from build123d import *

# Parameters (mm, degrees)
F2_SIZE  = 0.381
F4_DEPTH = 25.019
F5_R     = 6.875
F6_DEPTH = 25.781


with BuildPart() as f1:
    # F0 (on Front) → F1 (revolve)
    with BuildSketch(Plane.XZ):
        Polygon((22.225, 12.7), (-22.225, 12.7), (-22.225, 31.75), (-25.4, 31.75), (-25.4, 0), (25.4, 0), (25.4, 31.75), (22.225, 31.75), align=None)
    revolve(axis=Axis((0, 0, 0), (1, 0, 0)))

    # F2
    f2_edges = [f1.edges().sort_by_distance(p)[0] for p in [
        (-22.225, 0, -31.75),
        (-25.4, 0, -31.75),
        (22.225, 0, -31.75),
        (25.4, 0, -31.75),
    ]]
    chamfer(f2_edges, length=F2_SIZE)

    # F3 (on face) → F4 (cut)
    with BuildSketch(Plane.YZ.offset(25.4)):
        Polygon((6.35, -3.666174), (6.35, 3.666174), (0, 7.332348), (-6.35, 3.666174), (-6.35, -3.666174), (0, -7.332348), align=None)
    extrude(amount=-F4_DEPTH, mode=Mode.SUBTRACT)

    # F5 (on face) → F6 (cut)
    with BuildSketch(Plane(origin=(-25.4, 0, 0), x_dir=(0, -1, 0), z_dir=(-1, 0, 0))):
        Circle(F5_R)
    extrude(amount=-F6_DEPTH, mode=Mode.SUBTRACT)


solid = f1.part
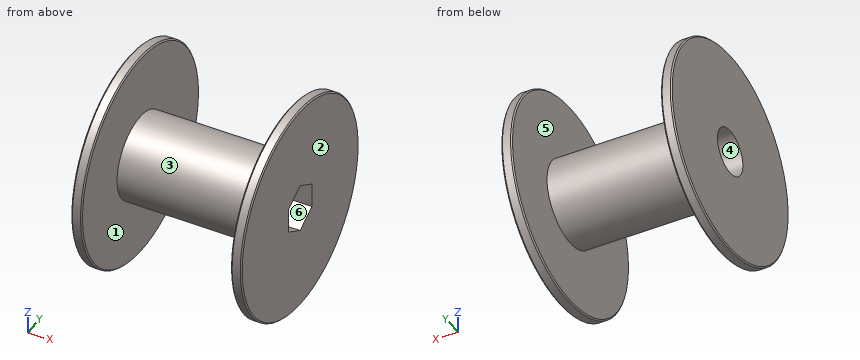
Geometry: final body of the model. Coordinates: model frame, mm. Face numbers are marked on the shaded views. A direction names the side the tool comes from. Round coordinates to 2 decimals unless told otherwise and drop trailing zeros. Order: outer loops, then holes, each group sorted by start corner. A loop starts at its lowest first (then second) coordinate and runs counter-clockwise, first axis right, second up. Notation, with made-up numbers: (15, 69) -> (67, 69) arc R27 ccw to (67, 95) -> close; hole circle Ø8 at (2.5, 38.25). An arc over 180 degrees is marked (long way). Put each result on its own line as item: value. Start each with the question number.
Q1. Line query: probe 1 along Y at (x, z) = (-7, 0) (3 decimals); probe 2 along X at (y, z) = (15, -2) (3 decimals). Output: solid intervals per line, ascending.
Q2. Section B-B on x = 13. Return the cut outline in (y, z), and give its area (3 significant figures).
Q3. First-contact query: pin 1 (8 mm diameter, centred on x = 14.5, y = -13.5, fed in from +Z); pin 2 (10 mm diameter, centred on x = -16.5, y = -6, fed in from +Z); pin 3 (2 mm diameter, centred on x = 8.5, z = 5.5, fed in from -Y). Flat tips, straight axial feed; report the tip coordinate or a pass-through.
Q4. Section C-C on x = -13.5. Return the cut outline in (y, z) (3 decimals).
Q5. Section A-A on z = 0. Return the cut outline in (x, y) (3 decimals), and give its area (3 significant figures).
Q6. Reachability of the marked faces 1 and 2 from +Z, -Z, +X, -X, +Y, -Y: full face, straight path, thin tool, end or side. Return the list, or none.
Q7. Pull-direction query (Z, two-part tool) for the marked faces 3, 4, 5 and 6; classes: +Z half, -Z half, draft (parallel to the pull), parting line (faces both ways), or undercut.
Ans:
1. probe 1: y = -12.7 to -6.875, 6.875 to 12.7
1. probe 2: x = -25.4 to -22.225, 22.225 to 25.4
2. outline: circle Ø25.4 at (0, 0); hole (-6.35, -3.67) -> (0, -7.33) -> (6.35, -3.67) -> (6.35, 3.67) -> (0, 7.33) -> (-6.35, 3.67) -> close
2. area: 367 mm2
3. pin 1: stops at z = 8.43
3. pin 2: stops at z = 12.66
3. pin 3: stops at y = -11.88
4. outline: circle Ø25.4 at (0, 0); hole circle Ø13.75 at (0, 0)
5. outline: (-25.4, -31.369) -> (-25.019, -31.75) -> (-22.606, -31.75) -> (-22.225, -31.369) -> (-22.225, -12.7) -> (22.225, -12.7) -> (22.225, -31.369) -> (22.606, -31.75) -> (25.019, -31.75) -> (25.4, -31.369) -> (25.4, -6.35) -> (0.381, -6.35) -> (0.381, -6.875) -> (-25.4, -6.875) -> close; (-25.4, 6.875) -> (0.381, 6.875) -> (0.381, 6.35) -> (25.4, 6.35) -> (25.4, 31.369) -> (25.019, 31.75) -> (22.606, 31.75) -> (22.225, 31.369) -> (22.225, 12.7) -> (-22.225, 12.7) -> (-22.225, 31.369) -> (-22.606, 31.75) -> (-25.019, 31.75) -> (-25.4, 31.369) -> close
5. area: 859 mm2
6. face 1: none
6. face 2: +Z, -Z, +X, +Y, -Y
7. face 3: parting line
7. face 4: undercut
7. face 5: draft
7. face 6: undercut
